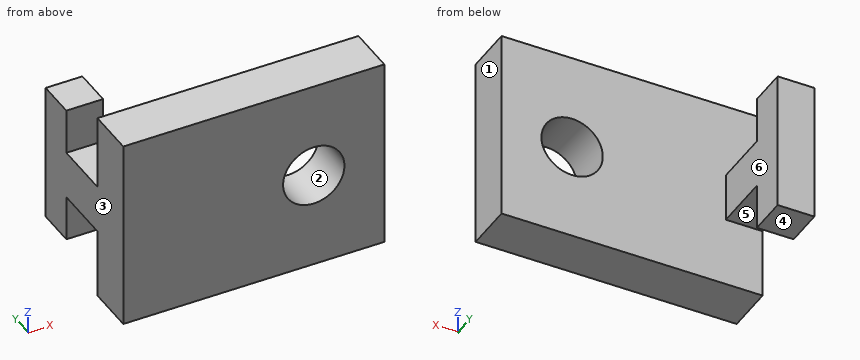
```python
from build123d import *

# Parameters (mm, degrees)
SKETCH1_W           = 685.8
SKETCH1_H           = 508
BOSS_EXTRUDE1_DEPTH = 127
SKETCH2_W           = 96.52
SKETCH2_H           = 127
BOSS_EXTRUDE2_DEPTH = 254
SKETCH3_W           = 96.52
SKETCH3_H           = 101.6
BOSS_EXTRUDE3_DEPTH = 120.65
SKETCH4_W           = 96.52
SKETCH4_H           = 101.6
BOSS_EXTRUDE4_DEPTH = 120.65
HOLE4_OUTLINE_R     = 80.645
HOLE4_DEPTH         = 127


# Read off the part's stored shape, not the designer's step: Hole4
with BuildPart() as part:
    # Sketch1 → Boss-Extrude1 (new body)
    with BuildSketch(Plane(origin=(0, 0, 0), x_dir=(1, 0, 0), z_dir=(0, 1, 0))):
        with Locations((342.9, 254)):
            Rectangle(SKETCH1_W, SKETCH1_H)
    extrude(amount=BOSS_EXTRUDE1_DEPTH)

    # Sketch2 → Boss-Extrude2 (add)
    with BuildSketch(Plane(origin=(0, 127, 0), x_dir=(1, 0, 0), z_dir=(0, 1, 0))):
        with Locations((48.26, 260.35)):
            Rectangle(SKETCH2_W, SKETCH2_H)
    extrude(amount=BOSS_EXTRUDE2_DEPTH)

    # Sketch3 → Boss-Extrude3 (add)
    with BuildSketch(Plane.XY.offset(-196.85)):
        with Locations((48.26, 330.2)):
            Rectangle(SKETCH3_W, SKETCH3_H)
    extrude(amount=BOSS_EXTRUDE3_DEPTH)

    # Sketch4 → Boss-Extrude4 (add)
    with BuildSketch(Plane(origin=(0, 0, -323.85), x_dir=(-1, 0, 0), z_dir=(0, 0, -1))):
        with Locations((-48.26, 330.2)):
            Rectangle(SKETCH4_W, SKETCH4_H)
    extrude(amount=BOSS_EXTRUDE4_DEPTH)

    # Hole4 outline → Hole4 (cut)
    with BuildSketch(Plane(origin=(0, 0, 0), x_dir=(1, 0, 0), z_dir=(0, 1, 0))):
        with Locations((500.38, 254)):
            Circle(HOLE4_OUTLINE_R)
    extrude(amount=HOLE4_DEPTH, mode=Mode.SUBTRACT)


solid = part.part
```
For this review, take the finished solid that the model builds, in its own axes (mm). Face numbers are marked on the shaded views. A direction names the side the tool comes from. Give positions to 0.01 mm unless a question says otherwise; leave off trailing zeros. Write each loop counter-clockwise with the first axis right and the second up, starting at its lowest first coordinate (ties: lowest second). Pieces come first, ordered by that corner, then holes.
Item 1: Take a section at B-B (z = -254). Give the boundary of the cut face in (x, y) (3 decimals).
Item 2: Take a section at A-A (x = 500.38). Give the boundary of the cut face in (y, z) (3 decimals).
Item 3: Take a section at D-D (x = 602). Give the boundary of the cut face in (y, z).
Item 4: Machinability: for the marked faces 4, 5 and 6, which of the approach directions +Z, -Z, +X, -X, +Y, -Y give a long, thin tool a straight path to every point of the face, cutting with its end or side? Answer none if there is none.
Item 5: The part is to be moulded in two halves that separate along X. For the marked faces 1, 2 and 3, say which applies: +X half, -X half, draft (parallel to the pull), parting line (faces both ways), or undercut.
Item 6: Take a section at C-C (y = 37). Give the boundary of the cut face in (x, z) (3 decimals), and give its area (3 significant figures).
Item 7: Wall thickness on probe 1 along Z at (x, y) = (500, 88); probe 2 along X at (y, z) = (99, -254) (3 decimals); probe 3 along Y at (x, z) = (426, -37): over which ranges is each line inside the solid? List them lowest first.
Item 8: Insertion check: P1, Ø12, axis at x = 199, z = -58, coming from the +Y side; P2, Ø1.5, axis at x = 76, y = 165, coming from the -Z side. Each pin has a flat end and moves straight along its axis. Give the tip position at first contact, or say it passes through.
Established:
1. outline: (0, 0) - (419.735, 0) - (419.735, 127) - (96.52, 127) - (96.52, 381) - (0, 381) - close; (581.025, 0) - (685.8, 0) - (685.8, 127) - (581.025, 127) - close
2. outline: (0, -508) - (127, -508) - (127, -334.645) - (0, -334.645) - close; (0, -173.355) - (127, -173.355) - (127, 0) - (0, 0) - close
3. outline: (0, -508) - (127, -508) - (127, 0) - (0, 0) - close
4. face 4: -Z, +X, -X, +Y
4. face 5: -Z, +X, -X
4. face 6: +Z, -Z, +X, +Y
5. face 1: +X half
5. face 2: undercut
5. face 3: -X half
6. outline: (0, -508) - (685.8, -508) - (685.8, 0) - (0, 0) - close; hole circle Ø161.29 at (500.38, -254)
6. area: 328,000 mm2
7. probe 1: z = -508 to -334.64, -173.36 to 0
7. probe 2: x = 0 to 419.735, 581.025 to 685.8
7. probe 3: y = 0 to 127
8. P1: stops at y = 127
8. P2: stops at z = -323.85
